```python
from build123d import *

# Parameters (mm, degrees)
SKETCH1_W               = 20.1
SKETCH1_H               = 4.2
BOSS_EXTRUDE1_DEPTH     = 4
SKETCH2_R               = 0.8
CUT_EXTRUDE1_DEPTH      = 4
LPATTERN2_COUNT         = 3
LPATTERN2_PITCH         = 15
MIRROR1_COPY_1_SKETCH_R = 0.8
MIRROR1_COPY_1_DEPTH    = 4
MIRROR1_COPY_2_SKETCH_R = 0.8
MIRROR1_COPY_2_DEPTH    = 4
SKETCH2_4_R             = 0.8
CUT_EXTRUDE3_DEPTH      = 4
LPATTERN3_COUNT         = 5
LPATTERN3_PITCH         = 30
SKETCH3_W               = 15
SKETCH3_H               = 6
CUT_EXTRUDE4_DEPTH      = 4


with BuildPart() as part:
    # Sketch1 → Boss-Extrude1 (new body)
    with BuildSketch(Plane.XY):
        Polygon((0, 15), (0, 67.5), (15.887452938, 67.5), (120, 19.2), (120, -4.2), (15.887452938, -52.5), (0, -52.5), (0, 0), (15, 0), (15, 15), align=None)
        with Locations((85.05, -2.1)):
            Rectangle(SKETCH1_W, SKETCH1_H, mode=Mode.SUBTRACT)
        with Locations((85.05, 17.1)):
            Rectangle(SKETCH1_W, SKETCH1_H, mode=Mode.SUBTRACT)
        with Locations((34.95, 17.1)):
            Rectangle(SKETCH1_W, SKETCH1_H, mode=Mode.SUBTRACT)
    extrude(amount=BOSS_EXTRUDE1_DEPTH)

    # Sketch2 → Cut-Extrude1 (cut)
    with BuildSketch(Plane.XY.offset(4)):
        with Locations((7.943726469, 57.5)):
            Circle(SKETCH2_R)
    cut_extrude1 = extrude(amount=-CUT_EXTRUDE1_DEPTH, mode=Mode.SUBTRACT)

    # LPattern2: Cut-Extrude1 ×3
    with Locations(*[(0, -i * LPATTERN2_PITCH, 0) for i in range(1, LPATTERN2_COUNT)]):
        add(cut_extrude1, mode=Mode.SUBTRACT)

    # Mirror1: Cut-Extrude1 across plane
    add(cut_extrude1.mirror(Plane.ZX.offset(7.5)), mode=Mode.SUBTRACT)

    # Mirror1 copy 1 sketch → Mirror1 copy 1 (cut)
    with BuildSketch(Plane(origin=(0, 30, 4), x_dir=(1, 0, 0), z_dir=(0, 0, 1))):
        with Locations((7.943726469, -57.5)):
            Circle(MIRROR1_COPY_1_SKETCH_R)
    extrude(amount=-MIRROR1_COPY_1_DEPTH, mode=Mode.SUBTRACT)

    # Mirror1 copy 2 sketch → Mirror1 copy 2 (cut)
    with BuildSketch(Plane(origin=(0, 45, 4), x_dir=(1, 0, 0), z_dir=(0, 0, 1))):
        with Locations((7.943726469, -57.5)):
            Circle(MIRROR1_COPY_2_SKETCH_R)
    extrude(amount=-MIRROR1_COPY_2_DEPTH, mode=Mode.SUBTRACT)

    # Sketch2_4 → Cut-Extrude3 (cut)
    with BuildSketch(Plane.XY.offset(4)):
        with Locations((110, 7.5)):
            Circle(SKETCH2_4_R)
    cut_extrude3 = extrude(amount=-CUT_EXTRUDE3_DEPTH, mode=Mode.SUBTRACT)

    # LPattern3: Cut-Extrude3 ×5
    with Locations(*[(-i * LPATTERN3_PITCH, 0, 0) for i in range(1, LPATTERN3_COUNT)]):
        add(cut_extrude3, mode=Mode.SUBTRACT)

    # Sketch3 → Cut-Extrude4 (cut)
    with BuildSketch(Plane.XY.offset(4)):
        with Locations((22.5, 7.5)):
            Rectangle(SKETCH3_W, SKETCH3_H)
    extrude(amount=-CUT_EXTRUDE4_DEPTH, mode=Mode.SUBTRACT)


solid = part.part
```
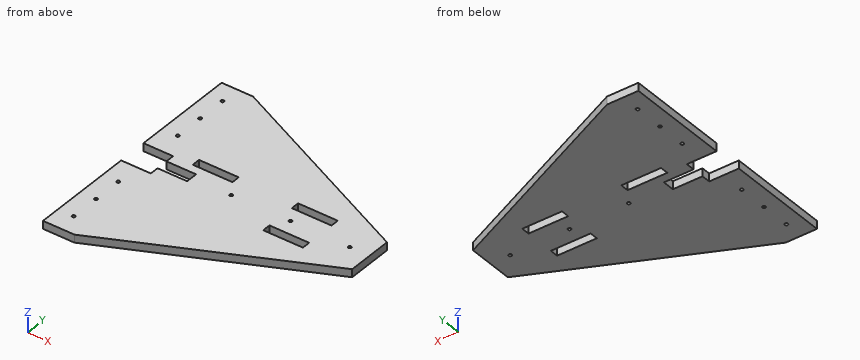
CAD build for the part. Positions are in the model's coordinates, mm. Round coordinates to 2 decimals unless told otherwise and drop trailing zeros. Order: outer loops, then holes, each group sorted by start corner. A loop starts at its lowest first (then second) coordinate and runs counter-clockwise, first axis right, second up.
Item 1: Probe line 1 along Y through (x, z) = (9.5, 0.3); line 2 along Y through (x, z) = (82.5, 2.3); line 3 along Y through (x, z) = (28, 2.15). List the from-to ranges inside material, lowest first.
Item 2: Saw through at C-C on y = 13. Write the cut outline in (x, z).
Item 3: Saw through at D-D on y = 25. Write the cut outline in (x, z).
Item 4: Saw through at A-A on x = 34.5. Write the cut outline in (y, z), then the cut area to 3 significant figures.
Item 5: Pin check, flat tip, straight feed: pin 1 (1.2 mm diameter, centred on x = 88, z = 2.5, fed in from -Y). Stop position of the tip, or through.
Item 6: Saw through at B-B on z = 1.45. State how many separate pieces and enclosed holes the cut face has, then the cut area to 4 significant figures.
Reported:
1. line 1: y = -52.5 to 0, 15 to 67.5
1. line 2: y = -21.6 to -4.2, 0 to 15, 19.2 to 36.6
1. line 3: y = -46.88 to 4.5, 10.5 to 15, 19.2 to 61.88
2. outline: (15, 0) - (120, 0) - (120, 4) - (15, 4) - close
3. outline: (0, 0) - (107.5, 0) - (107.5, 4) - (0, 4) - close
4. outline: (-43.87, 0) - (15, 0) - (15, 4) - (-43.87, 4) - close; (19.2, 0) - (58.87, 0) - (58.87, 4) - (19.2, 4) - close
4. area: 394 mm2
5. pin 1: stops at y = -19.32
6. separate pieces: 1
6. enclosed holes: 12
6. area: 8,785 mm2
